Here's how the part is built. I have some questions about the finished solid (model axes, mm). Face numbers are marked on the shaded views. Coordinates: 2 decimals unless noted, no trailing zeros. Write each loop counter-clockwise with the first axis right and the second up, starting at its lowest first coordinate (ties: lowest second). Pieces come first, ordered by that corner, then holes.
Item 1: I want a section at A-A (y = 72.5). Please give me the cut outline in (x, z), and give its area (3 significant figures).
Item 2: Please list where this line runs through material, in increasing order: line 1 (Y direction, x = 45, z = 14).
Item 3: I want a section at C-C (x = -52). Please give me the cut outline in (y, z), and give its area (3 significant figures).
Item 4: If we mould it in two halves opening along X, with no side actions, what happens to the marked faces 1, 2 and 3? For each: pulls with the +X half, pulls with the -X half, needs draft (parallel to the pull), parting line crosses it, or undercut.
Item 5: I'm going to push flat-ended pins straight in: P1, Ø12.5, axis at x = 57, z = 31, coming from the +Y side; P2, Ø1, axis at x = 65.5, y = 67.5, coming from the +Z side; P3, Ø0.6, axis at x = -65, z = 24, coming from the +Y side. Where does each tip first touch, or does it pass through?
Item 6: I want a section at B-B (z = 22). Please give me the cut outline in (x, y), and give its area (3 significant figures).
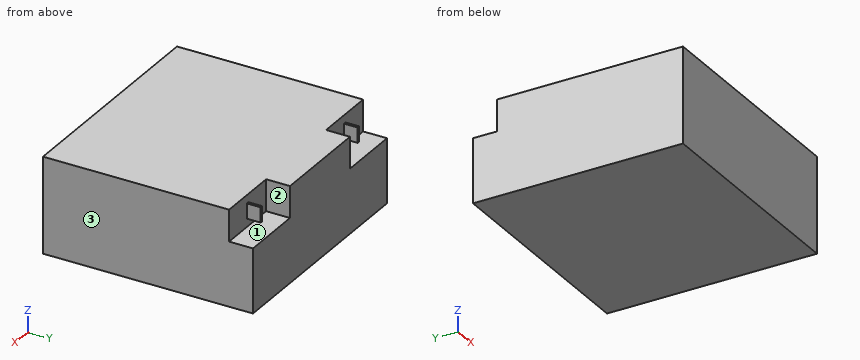
from build123d import *

# Parameters (mm, degrees)
SKETCH1_W           = 181
SKETCH1_H           = 167
BOSS_EXTRUDE1_DEPTH = 38
SKETCH3_W           = 50
SKETCH3_H           = 19
CUT_EXTRUDE1_DEPTH  = 25
SKETCH4_W           = 2
SKETCH4_H           = 12
BOSS_EXTRUDE2_DEPTH = 11


with BuildPart() as part:
    # Sketch1 → Boss-Extrude1 (new body, symmetric)
    with BuildSketch(Plane.XY):
        Rectangle(SKETCH1_W, SKETCH1_H)
    extrude(amount=BOSS_EXTRUDE1_DEPTH, both=True)

    # Sketch3 → Cut-Extrude1 (cut)
    with BuildSketch(Plane.XY.offset(38)):
        with Locations((-65.5, 74)):
            Rectangle(SKETCH3_W, SKETCH3_H)
        with Locations((65.5, 74)):
            Rectangle(SKETCH3_W, SKETCH3_H)
    extrude(amount=-CUT_EXTRUDE1_DEPTH, mode=Mode.SUBTRACT)

    # Sketch4 → Boss-Extrude2 (add)
    with BuildSketch(Plane(origin=(0, 64.5, 0), x_dir=(1, 0, 0), z_dir=(0, 1, 0))):
        with Locations((-65.5, -25.5)):
            Rectangle(SKETCH4_W, SKETCH4_H)
        with Locations((65.5, -25.5)):
            Rectangle(SKETCH4_W, SKETCH4_H)
    extrude(amount=BOSS_EXTRUDE2_DEPTH)


solid = part.part
Answer:
1. outline: (-90.5, -38) - (90.5, -38) - (90.5, 13) - (40.5, 13) - (40.5, 38) - (-40.5, 38) - (-40.5, 13) - (-90.5, 13) - close; (-66.5, 19.5) - (-64.5, 19.5) - (-64.5, 31.5) - (-66.5, 31.5) - close; (64.5, 19.5) - (66.5, 19.5) - (66.5, 31.5) - (64.5, 31.5) - close
1. area: 11,300 mm2
2. line 1: y = -83.5 to 64.5
3. outline: (-83.5, -38) - (83.5, -38) - (83.5, 13) - (64.5, 13) - (64.5, 38) - (-83.5, 38) - close
3. area: 12,200 mm2
4. face 1: needs draft
4. face 2: undercut
4. face 3: pulls with the +X half
5. P1: stops at y = 64.5
5. P2: stops at z = 31.5
5. P3: stops at y = 75.5
6. outline: (-90.5, -83.5) - (90.5, -83.5) - (90.5, 64.5) - (66.5, 64.5) - (66.5, 75.5) - (64.5, 75.5) - (64.5, 64.5) - (40.5, 64.5) - (40.5, 83.5) - (-40.5, 83.5) - (-40.5, 64.5) - (-64.5, 64.5) - (-64.5, 75.5) - (-66.5, 75.5) - (-66.5, 64.5) - (-90.5, 64.5) - close
6. area: 28,400 mm2
